Input: part model. Units: mm. Frame: model coordinates. Give positions to 0.01 mm unless a question says otherwise; leave off trailing zeros. Write each loop counter-clockwise with the first axis right and the second up, starting at its lowest first coordinate (ties: lowest second). Pieces come first, ordered by that corner, then holes. Notation, with made-up numbers: (61.25, 47) -> (90.25, 47) arc R22 cw to (90.25, 59) -> close; hole circle Ø1 at (-4, -12). An arc over 180 degrees is marked (long way). Answer as a JSON object with one key per item and string values. Group by question number.
from build123d import *

# Parameters (mm, degrees)
F1_DEPTH = 2.9718


with BuildPart() as f1:
    # F0 (on Front) → F1 (new body)
    with BuildSketch(Plane.XZ):
        with BuildLine():
            Line((135.1153, -60.5282), (152.4, -60.5282))
            Line((152.4, -60.5282), (152.4, -38.1))
            Line((152.4, -38.1), (149.4282, -38.1))
            Line((149.4282, -38.1), (149.4282, -27.1653))
            Line((149.4282, -27.1653), (139.2682, -27.1653))
            Line((139.2682, -27.1653), (139.2682, -29.2862))
            Line((139.2682, -29.2862), (136.6266, -29.2862))
            Line((136.6266, -29.2862), (136.6266, -27.1653))
            Line((136.6266, -27.1653), (131.5974, -27.1653))
            Line((131.5974, -27.1653), (131.5974, -23.6347))
            Line((131.5974, -23.6347), (136.6266, -23.6347))
            Line((136.6266, -23.6347), (136.6266, -21.5138))
            Line((136.6266, -21.5138), (139.2682, -21.5138))
            Line((139.2682, -21.5138), (139.2682, -23.6347))
            Line((139.2682, -23.6347), (149.4282, -23.6347))
            Line((149.4282, -23.6347), (149.4282, -12.7))
            Line((149.4282, -12.7), (152.4, -12.7))
            Line((152.4, -12.7), (152.4, -1.771027))
            ThreePointArc((152.4, -1.771027), (150.877363, 4.258612), (146.674559, 8.842433))
            Line((146.674559, 8.842433), (66.67517, 61.41346))
            ThreePointArc((66.67517, 61.41346), (63.340602, 62.967188), (59.700611, 63.5))
            Line((59.700611, 63.5), (-139.7, 63.5))
            ThreePointArc((-139.7, 63.5), (-148.680256, 59.780256), (-152.4, 50.8))
            Line((-152.4, 50.8), (-152.4, 35.369483))
            ThreePointArc((-152.4, 35.369483), (-149.689715, 27.52757), (-142.715654, 23.032715))
            Line((-142.715654, 23.032715), (-44.337678, -1.015234))
            ThreePointArc((-44.337678, -1.015234), (-39.095537, -3.703229), (-35.630256, -8.467386))
            Line((-35.630256, -8.467386), (-3.751196, -57.696563))
            ThreePointArc((-3.751196, -57.696563), (0.838391, -61.948701), (6.901284, -63.493472))
            Line((6.901284, -63.493472), (17.805659, -63.5))
            ThreePointArc((17.805659, -63.5), (19.05, -60.452), (20.294341, -63.5))
            Line((20.294341, -63.5), (38.1, -63.5))
            Line((38.1, -63.5), (38.1, -60.5282))
            Line((38.1, -60.5282), (55.3847, -60.5282))
            Line((55.3847, -60.5282), (55.3847, -50.3682))
            Line((55.3847, -50.3682), (53.2638, -50.3682))
            Line((53.2638, -50.3682), (53.2638, -47.7266))
            Line((53.2638, -47.7266), (55.3847, -47.7266))
            Line((55.3847, -47.7266), (55.3847, -42.6974))
            Line((55.3847, -42.6974), (58.9153, -42.6974))
            Line((58.9153, -42.6974), (58.9153, -47.7266))
            Line((58.9153, -47.7266), (61.0362, -47.7266))
            Line((61.0362, -47.7266), (61.0362, -50.3682))
            Line((61.0362, -50.3682), (58.9153, -50.3682))
            Line((58.9153, -50.3682), (58.9153, -60.5282))
            Line((58.9153, -60.5282), (76.2, -60.5282))
            Line((76.2, -60.5282), (76.2, -63.5))
            Line((76.2, -63.5), (94.005659, -63.5))
            ThreePointArc((94.005659, -63.5), (95.25, -60.452), (96.494341, -63.5))
            Line((96.494341, -63.5), (114.3, -63.5))
            Line((114.3, -63.5), (114.3, -60.5282))
            Line((114.3, -60.5282), (131.5847, -60.5282))
            Line((131.5847, -60.5282), (131.5847, -50.3682))
            Line((131.5847, -50.3682), (129.4638, -50.3682))
            Line((129.4638, -50.3682), (129.4638, -47.7266))
            Line((129.4638, -47.7266), (131.5847, -47.7266))
            Line((131.5847, -47.7266), (131.5847, -42.6974))
            Line((131.5847, -42.6974), (135.1153, -42.6974))
            Line((135.1153, -42.6974), (135.1153, -47.7266))
            Line((135.1153, -47.7266), (137.2362, -47.7266))
            Line((137.2362, -47.7266), (137.2362, -50.3682))
            Line((137.2362, -50.3682), (135.1153, -50.3682))
            Line((135.1153, -50.3682), (135.1153, -60.5282))
        make_face()
        Polygon((-31.988177, 34.010913), (-33.004593, 31.218334), (-42.55187, 34.693259), (-41.535454, 37.485837), align=None, mode=Mode.SUBTRACT)
        Polygon((20.521846, 14.898827), (19.505431, 12.106248), (9.958154, 15.581173), (10.974569, 18.373752), align=None, mode=Mode.SUBTRACT)
    extrude(amount=F1_DEPTH)


solid = f1.part
1. Contact query for flat-ended pins moving along their axis: pin 1 Ø0.9 at (y, z) = (-2, -45) entering from -X; pin 2 Ø1.1 at (x, y) = (131, -1.5) entering from +Z; pin 3 Ø1.7 at (y, z) = (-1, -28.5) entering from -X. Output: stop coordinate, or through.
2. Section C-C (x = 108.5). Return the cut outline in (y, z).
3. Line query: line 1 (X direction, y = -1.05, z = -62.23); line 2 (X direction, y = -0.45, z = -50); line 3 (Z direction, x = 95.25, y = -2.3). Output: solid intervals per line, ascending.
4. Section A-A (y = -2.35). State how many separate pieces and enclosed holes the cut face has, plus the area to 3 significant figures.
5. Section B-B (x = -73). Return the cut outline in (y, z), plus the area to 3 significant figures.
Working result:
{
 "1": {"pin 1": "stops at x = -12.26", "pin 2": "stops at z = 19.5", "pin 3": "stops at x = -23.21"},
 "2": {"outline": "(-2.97, -63.5) -> (0, -63.5) -> (0, 33.93) -> (-2.97, 33.93) -> close"},
 "3": {"line 1": "x = 1.39 to 17.27, 20.83 to 38.1, 76.2 to 93.47, 97.03 to 114.3", "line 2": "x = -8.74 to 53.26, 61.04 to 129.46, 137.24 to 152.4", "line 3": "z = -60.45 to 42.64"},
 "4": {"separate pieces": "1", "enclosed holes": "2", "area": "25,800 mm^2"},
 "5": {"outline": "(-2.97, 5.99) -> (0, 5.99) -> (0, 63.5) -> (-2.97, 63.5) -> close", "area": "171 mm^2"}
}
